from build123d import *

# Parameters (mm, degrees)
F0_R     = 63.5
F1_DEPTH = 127
F1_TAPER = -20
F2_R     = 25.4
F4_T     = -12.7


# Not quite as in the source:
# - a fillet or chamfer that OpenCascade refuses, or shapes differently, is made with other operations: its cross-section is extruded or revolved along the edge and cut away or added


with BuildPart() as f1:
    # F0 (on Front) → F1 (new body, symmetric)
    with BuildSketch(Plane.XZ):
        Circle(F0_R)
    extrude(amount=F1_DEPTH, both=True, taper=F1_TAPER)

    # F2
    f2_edges = [f1.edges().sort_by_distance(p)[0] for p in [
        (-63.5, 0, 0),
        (-109.72422, 127, 0),
    ]]
    fillet(f2_edges, radius=F2_R)

    # F3: chamfer of 63.5 on 1 edges, made by hand

    # F3_s1 → F3_t2 (revolve, cut)
    with BuildSketch(Plane.XY):
        Polygon((88.0059406506, -67.3295185801), (46.2242197518, -127), (109.7242197518, -127), align=None)
    revolve(axis=Axis((0, -127, 0), (0, 1, 0)), mode=Mode.SUBTRACT)

    # F4
    f4_openings = [f1.faces().sort_by_distance(p)[0] for p in [
        (0, -127, 0),
    ]]
    offset(amount=F4_T, openings=f4_openings)


solid = f1.part
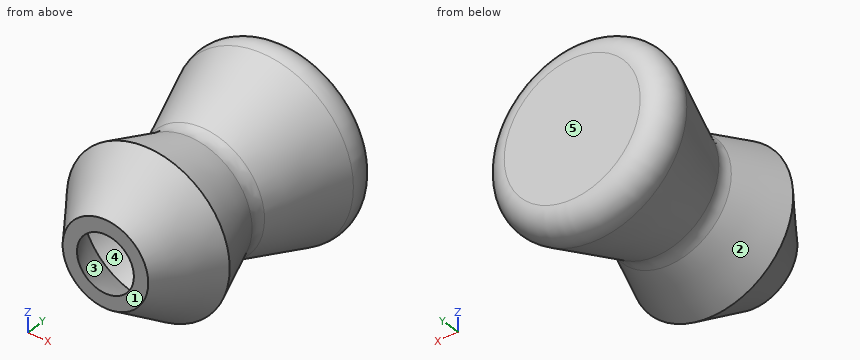
Build history of the part. All positions in model axes, mm. Face numbers are marked on the shaded views. A direction names the side the tool comes from. Round coordinates to 2 decimals unless told otherwise and drop trailing zeros. Write each loop counter-clockwise with the first axis right and the second up, starting at its lowest first coordinate (ties: lowest second). Pieces come first, ordered by that corner, then holes. Notation, with made-up numbers: (-21.5, 39.5) - (17.5, 39.5) arc R14 cw to (17.5, 54.5) - close; hole circle Ø8 at (-30.5, 74.25). An arc over 180 degrees is marked (long way). One line per question, with ' | ' between items.
1. Band-saw the part on C-C, the plane y = 103.5. Write the cut outline in (x, z), and give its area (3 significant figures).
Results are:
outline: circle Ø197.56 at (0, 0); hole circle Ø172.01 at (0, 0) | area: 7,410 mm^2
2. Mould opens along X. For the marked faces 1, 2 and 3 say: released by +X, released by -X, zero draft, split by the parting line, or undercut.
Results are:
face 1: zero draft | face 2: split by the parting line | face 3: undercut
3. Tool access for the marked faces 4 and 5: list every direction of +Z, -Z, +X, -X, +Y, -Y with a clear straight run to the whole face (end or side of a thin tool).
Results are:
face 4: none | face 5: +Z, -Z, +X, -X, +Y
4. Band-saw the part on A-A, the plane z = 79. Give the number of separate pieces and of enclosed holes in the cut face, and give its area (3 significant figures).
Results are:
separate pieces: 2 | enclosed holes: 1 | area: 7,450 mm^2
5. Drop flat-ended pins along their axis: pin 1 Ø10 at (y, z) = (46.5, 78) entering from -X; pin 2 Ø4 at (y, z) = (-47, 70) entering from -X; pin 3 Ø6 at (y, z) = (27.5, 66.5) entering from -X. Give the stop position or say it passes through.
Results are:
pin 1: x = -34.58 | pin 2: x = -43.56 | pin 3: x = -37.47
6. Drill centre lines: line 1 along Y through (x, z) = (35.5, -57); line 2 along Y through (x, z) = (39, -66); line 3 along Y through (x, z) = (-66, -38.5). Where is each one in solid material? Low to high. Write a range as from..to.
Results are:
line 1: -97.11..-74.97, -47.16..-10.03, 10.03..47.16, 114.3..127 | line 2: -83.53..-36.16, 36.16..73.29, 113.89..126.8 | line 3: -83.89..-35.47, 35.47..72.6, 113.95..126.83
